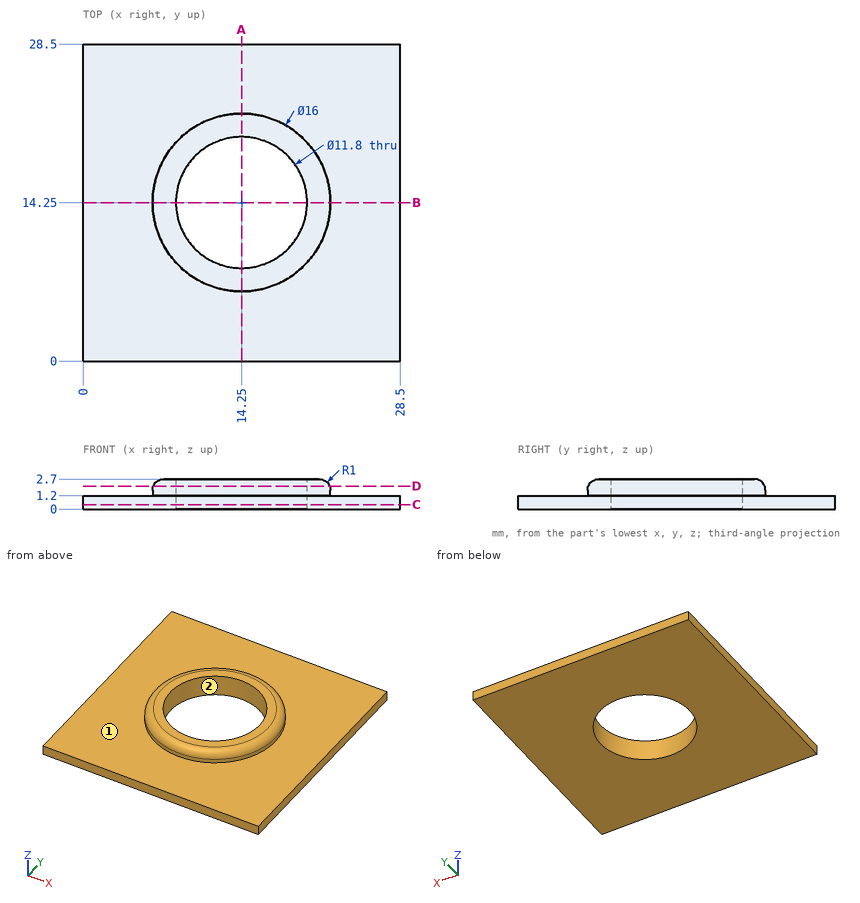
Part print with two shaded views. Sizes in mm from the minimum x, y, z corner. Coordinates: 2 decimals unless noted, no trailing zeros. Write each loop counter-clockwise with the first axis right and the second up, starting at its lowest first coordinate (ties: lowest second). Pieces come first, ordered by that corner, then holes.
(1) Cut at D-D on z = 2.05. List the corners of the cut face in (x, y), and give its area (3 significant figures).
(2) Mould opens along Y. For the marked faces 1 and 2 say: pulls with the +Y half, pulls with the -Y half, needs draft (parallel to the pull), parting line crosses it, or undercut.
(3) Cut at C-C on z = 0.4. List the corners of the cut face in (x, y), and give its area (3 significant figures).
(4) Cut at A-A on x = 14.25. List the corners of the cut face in (y, z).
(5) Drill centre lines: line 1 (Y direction, x = 14.25, z = 1.15); line 2 (Y direction, x = 14.25, z = 1.8); line 3 (Z direction, x = 6, y = 24.25). Where is each one in solid material? Low to high.
(6) Pin check, flat tip, straight feed: pin 1 Ø12 at (x, y) = (9.5, 14.5) entering from -Z. Stop position of the tip, or through.
Working result:
1. outline: circle Ø15.87 at (14.25, 14.25); hole circle Ø11.8 at (14.25, 14.25)
1. area: 88.5 mm2
2. face 1: needs draft
2. face 2: undercut
3. outline: (0, 0) - (28.5, 0) - (28.5, 28.5) - (0, 28.5) - close; hole circle Ø11.8 at (14.25, 14.25)
3. area: 703 mm2
4. outline: (0, 0) - (8.35, 0) - (8.35, 2.7) - (7.25, 2.7) arc R1 ccw to (6.25, 1.7) - (6.25, 1.2) - (0, 1.2) - close; (20.15, 0) - (28.5, 0) - (28.5, 1.2) - (22.25, 1.2) - (22.25, 1.7) arc R1 ccw to (21.25, 2.7) - (20.15, 2.7) - close
5. line 1: y = 0 to 8.35, 20.15 to 28.5
5. line 2: y = 6.26 to 8.35, 20.15 to 22.24
5. line 3: z = 0 to 1.2
6. pin 1: stops at z = 0
